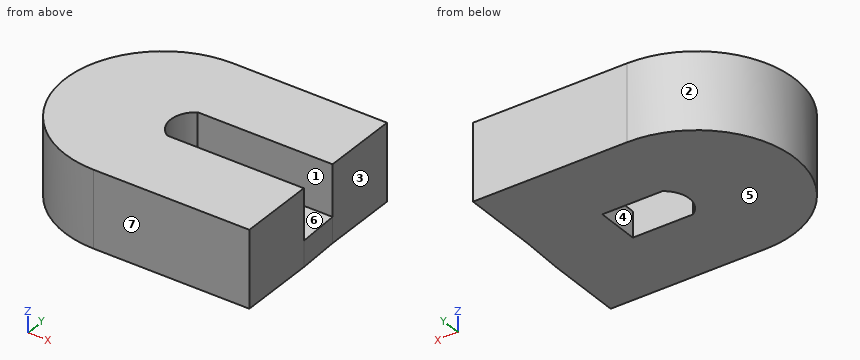
```python
from build123d import *

# Parameters (mm, degrees)
BOSS_EXTRUDE1_DEPTH = 6
BOSS_EXTRUDE2_DEPTH = 2


with BuildPart() as part:
    # Sketch1 → Boss-Extrude1 (new body)
    with BuildSketch(Plane.XY):
        with BuildLine():
            Line((-2, 6.705426357), (2, 6.705426357))
            Line((2, 6.705426357), (8.562541674, 6.705426357))
            Line((8.562541674, 6.705426357), (8.562541674, 12.705426357))
            Line((8.562541674, 12.705426357), (3.5, 12.705426357))
            Line((3.5, 12.705426357), (-3.5, 12.705426357))
            ThreePointArc((-3.5, 12.705426357), (-11.18, 5.025426357), (-3.5, -2.654573643))
            Line((-3.5, -2.654573643), (3.5, -2.654573643))
            Line((3.5, -2.654573643), (8.700403781, -2.654573643))
            Line((8.700403781, -2.654573643), (8.700403781, 3.345426357))
            Line((8.700403781, 3.345426357), (2, 3.345426357))
            Line((2, 3.345426357), (-2, 3.345426357))
            ThreePointArc((-2, 3.345426357), (-2.914827203, 5.025426357), (-2, 6.705426357))
        make_face()
    extrude(amount=BOSS_EXTRUDE1_DEPTH)

    # Sketch2 → Boss-Extrude2 (add)
    with BuildSketch(Plane.XY):
        Polygon((8.562541674, 6.705426357), (8.700403781, 3.345426357), (2.7, 3.345426357), (2.7, 6.705426357), align=None)
    extrude(amount=BOSS_EXTRUDE2_DEPTH)


solid = part.part
```
Verification items for the finished model (mm, model axes). Face numbers are marked on the shaded views. A direction names the side the tool comes from. Give positions to 0.01 mm unless a question says otherwise; leave off trailing zeros. Write each loop counter-clockwise with the first axis right and the second up, starting at its lowest first coordinate (ties: lowest second). Pieces come first, ordered by that corner, then holes. Notation, with made-up numbers: M 26.25,26.25 L 83.25,26.25 A13 ccw 83.25,38.25 Z; hole C 4,88.5 d6. An arc over 180 degrees is marked long. One line per question, with ' | ' between items.
1) Set-up check for the marked faces 1, 2, 3 and 4: record each of +Z, -Z, +X, -X, +Y, -Y from which the full face is reachable in a straight line by a thin tool's end or side.
Result:
face 1: +Z | face 2: +Z, -Z, -X | face 3: +Z, -Z, +X, +Y | face 4: +Z, -Z
2) Section check C-C on x = 6.25. Enter the section's corners in (y, z), plus the area to 3 significant figures.
Result:
outline: M -2.65,0 L 12.71,0 L 12.71,6 L 6.71,6 L 6.71,2 L 3.35,2 L 3.35,6 L -2.65,6 Z | area: 78.7 mm2
3) Mould release check, pull along Y, two halves, no side actions. Record for the marked faces 5, 6 and 7: released by +Y, released by -Y, zero draft, split by the parting line, or undercut.
Result:
face 5: zero draft | face 6: undercut | face 7: released by -Y
4) Section check B-B on x = 0.5. Enter the section's corners in (y, z), plus the area to 3 significant figures.
Result:
outline: M -2.65,0 L 3.35,0 L 3.35,6 L -2.65,6 Z; M 6.71,0 L 12.71,0 L 12.71,6 L 6.71,6 Z | area: 72.0 mm2
5) Gauge pin test, flat ends, axial feed: pin 1 Ø3 at (y, z) = (4.5, 3.5) entering from -X; pin 2 Ø3 at (y, z) = (8.5, 3.5) entering from +X; pin 3 Ø2 at (y, z) = (8.5, 2) entering from -X; pin 4 Ø2 at (x, y) = (-0.5, 5) entering from -Z. Record the tip position at first contact, or that the pin passes through.
Result:
pin 1: stops at x = -11.18 | pin 2: stops at x = 8.56 | pin 3: stops at x = -10.77 | pin 4: passes through
6) Section check A-A on z = 0.65. Enter the section's corners in (x, y), plus the area to 3 significant figures.
Result:
outline: M -3.5,-2.65 L 8.7,-2.65 L 8.7,3.35 L 8.56,6.71 L 8.56,12.71 L -3.5,12.71 A7.68 ccw Z; hole M -2,3.35 L 2.7,3.35 L 2.7,6.71 L -2,6.71 A2 ccw Z | area: 261 mm2
7) Section check D-D on z = 3.75. Enter the section's corners in (x, y).
Result:
outline: M -3.5,-2.65 L 8.7,-2.65 L 8.7,3.35 L -2,3.35 A2 cw -2,6.71 L 8.56,6.71 L 8.56,12.71 L -3.5,12.71 A7.68 ccw Z
8) Thickness scan on line 1 along Y through (x, z) = (-0.25, 0.9); line 2 along X through (y, z) = (5, 0.7); line 3 along X through (y, z) = (-1.5, 2.05). Record the ranges inside material, lowest first. Write a range as [from, to].
Result:
line 1: y = [-2.65, 3.35], [6.71, 12.71] | line 2: x = [-11.18, -2.91], [2.7, 8.63] | line 3: x = [-7.55, 8.7]
